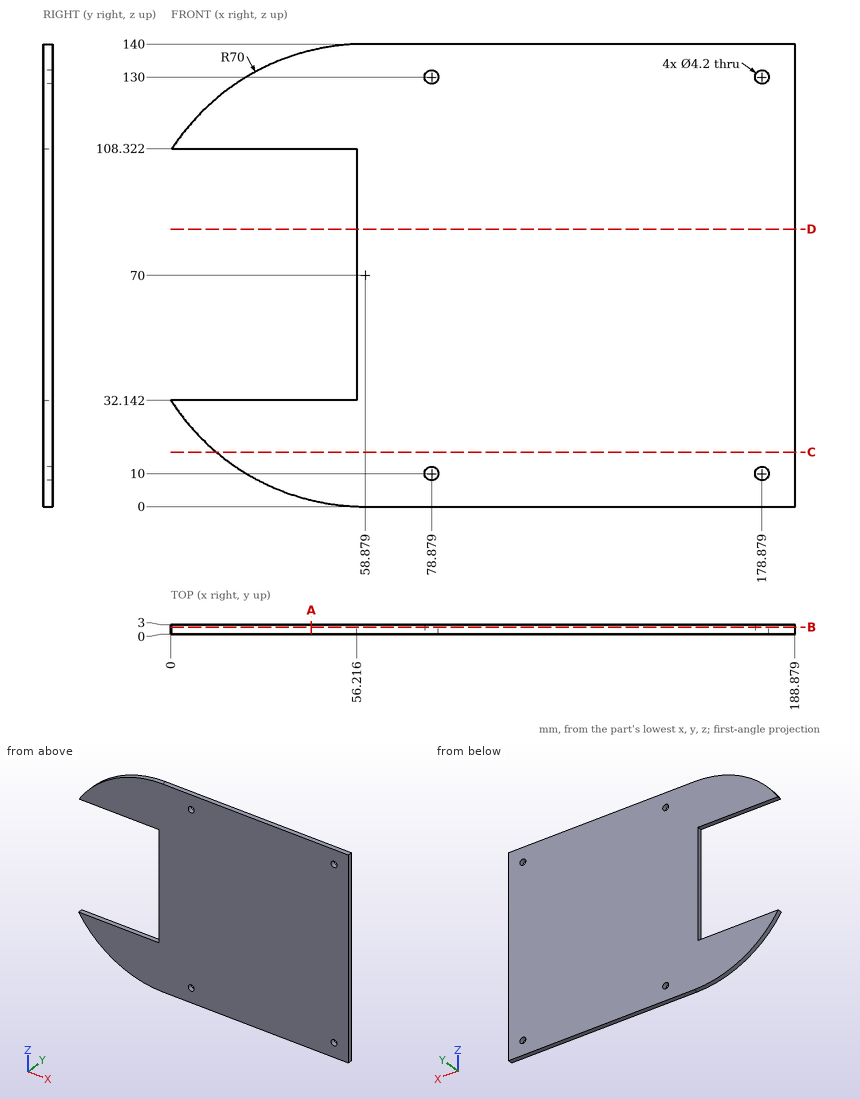
Check sheet for the drawn part. Datum: minimum x, y, z corner. Units: mm. Give positions to 0.01 mm unless a question says otherwise; leave off trailing zeros. Order: outer loops, then holes, each group sorted by start corner. A loop starts at its lowest first (then second) coordinate and runs counter-clockwise, first axis right, second up. Notation, with made-up numbers: (-30.5, -18.75) - (-9.5, -18.75) arc R33 cw to (-9.5, 14.25) - close; hole circle Ø7 at (87.25, 51.25). An arc over 180 degrees is marked (long way). Answer as a JSON object with one key per item and string values.
(1) Cross-section at C-C (z = 16.5). Record the cut outline in (x, y).
Report:
{"outline": "(13.74, 0) - (188.88, 0) - (188.88, 3) - (13.74, 3) - close"}
(2) Cross-section at B-B (y = 2.2). Record the cut outline in (x, z) (1 decimal).
Report:
{"outline": "(0, 32.1) arc R70 ccw to (58.9, 0) - (188.9, 0) - (188.9, 140) - (58.9, 140) arc R70 ccw to (0.3, 108.3) - (56.2, 108.3) - (56.2, 32.1) - close; hole circle Ø4.2 at (78.9, 10); hole circle Ø4.2 at (78.9, 130); hole circle Ø4.2 at (178.9, 10); hole circle Ø4.2 at (178.9, 130)"}
(3) Material ranges on line 1 (Z direction, x = 77.5, y = 0.6) (1 decimal); line 2 (X direction, y = 0.5, z = 42.5) (1 decimal); line 3 (X direction, y = 1.15, z = 116.5) (1 decimal), recorded low to high.
Report:
{"line 1": "0 to 8.4, 11.6 to 128.4, 131.6 to 140", "line 2": "56.2 to 188.9", "line 3": "6.6 to 188.9"}
(4) Depth check by flat-ended pin: pin 1 Ø0.9 at (x, y) = (17, 1.5) entering from +Z (1 decimal); pin 2 Ø0.9 at (y, z) = (1, 53.5) entering from -X (1 decimal); pin 3 Ø4 at (x, z) = (178.88, 130) entering from -Y. Enter the tip coordinate at first touch or a pass-through.
Report:
{"pin 1": "z = 126.4", "pin 2": "x = 56.2", "pin 3": "through"}
(5) Cross-section at D-D (z = 84). Record the cut outline in (x, y) (1 decimal), then the cut area to 3 significant figures.
Report:
{"outline": "(56.2, 0) - (188.9, 0) - (188.9, 3) - (56.2, 3) - close", "area": "398 mm^2"}
(6) Cross-section at A-A (x = 42.5). Record the cut outline in (y, z).
Report:
{"outline": "(0, 1.94) - (3, 1.94) - (3, 32.14) - (0, 32.14) - close; (0, 108.32) - (3, 108.32) - (3, 138.06) - (0, 138.06) - close"}
